from build123d import *

# Parameters (mm, degrees)
SALIENTE_EXTRUIR1_DEPTH = 5
CROQUIS2_R              = 7.5
CORTAR_EXTRUIR1_DEPTH   = 6


with BuildPart() as part:
    # Croquis1 → Saliente-Extruir1 (new body)
    with BuildSketch(Plane(origin=(0, 0, 0), x_dir=(1, 0, 0), z_dir=(0, 1, 0))):
        with BuildLine():
            Line((-6, -10), (6, -10))
            ThreePointArc((6, -10), (8.828427125, -8.828427125), (10, -6))
            Line((10, -6), (10, 6))
            ThreePointArc((10, 6), (8.828427125, 8.828427125), (6, 10))
            Line((6, 10), (-6, 10))
            ThreePointArc((-6, 10), (-8.828427125, 8.828427125), (-10, 6))
            Line((-10, 6), (-10, -6))
            ThreePointArc((-10, -6), (-8.828427125, -8.828427125), (-6, -10))
        make_face()
    extrude(amount=SALIENTE_EXTRUIR1_DEPTH)

    # Croquis2 → Cortar-Extruir1 (cut, through all)
    with BuildSketch(Plane(origin=(0, 5, 0), x_dir=(1, 0, 0), z_dir=(0, 1, 0))):
        Circle(CROQUIS2_R)
    extrude(amount=-CORTAR_EXTRUIR1_DEPTH, mode=Mode.SUBTRACT)


solid = part.part
Verification items for the finished model (mm, model axes). Coordinates: 2 decimals unless noted, no trailing zeros. Order: outer loops, then holes, each group sorted by start corner. A loop starts at its lowest first (then second) coordinate and runs counter-clockwise, first axis right, second up.
1. Scan lines: line 1 (Z direction, x = 0, y = 3.9); line 2 (Z direction, x = -3, y = 0.6). Record each from-to range of solid material in increasing order.
Results found:
line 1: z = -10 to -7.5, 7.5 to 10
line 2: z = -10 to -6.87, 6.87 to 10
2. Sectioned sample at A-A, the plane y = 2.5. Record the cut outline in (x, z), and give its area (3 significant figures).
Results found:
outline: (-10, -6) arc R4 ccw to (-6, -10) - (6, -10) arc R4 ccw to (10, -6) - (10, 6) arc R4 ccw to (6, 10) - (-6, 10) arc R4 ccw to (-10, 6) - close; hole circle Ø15 at (0, 0)
area: 210 mm2
3. Sectioned sample at B-B, the plane z = 0. Record the cut outline in (x, y), and give its area (3 significant figures).
Results found:
outline: (-10, 0) - (-7.5, 0) - (-7.5, 5) - (-10, 5) - close; (7.5, 0) - (10, 0) - (10, 5) - (7.5, 5) - close
area: 25.0 mm2
4. Sectioned sample at C-C, the plane x = 0. Record the cut outline in (y, z), and give its area (3 significant figures).
Results found:
outline: (0, -10) - (5, -10) - (5, -7.5) - (0, -7.5) - close; (0, 7.5) - (5, 7.5) - (5, 10) - (0, 10) - close
area: 25.0 mm2
5. Go/stop test with a flat-tipped pin: pin 1 Ø1.5 at (y, z) = (1, 8) entering from +X. Record where the tip stops, or that it passes through.
Results found:
pin 1: stops at x = 9.8
6. Release check for a two-part mould opening along X. For faces 1 (the face through (0, 2, -10)), 2 (the face through (-10, 2, 0)), 3 (the face through (-7.493, 2.535, -0.33)), 4 (the face through (8.797, 2.465, 8.859)) record: +X half, -X half, draft (parallel to the pull), parting line (faces both ways), or undercut.
Results found:
face 1: draft
face 2: -X half
face 3: undercut
face 4: +X half
